Model file for the job. Use its own axes, mm. A direction names the side the tool comes from. Give positions to 0.01 mm unless a question says otherwise; leave off trailing zeros. Loops run counter-clockwise (first coordinate to the right, second up) from the corner with the lowest first, then second, coordinate; pieces in that order, holes last. Notation, with made-up numbers: M -33.75,23.25 L 7.25,23.25 A10 cw 7.25,36.25 Z; hole C 27.5,49 d4. An arc over 180 degrees is marked long. Answer in a Markdown table with one row per item.
```python
from build123d import *

# Parameters (mm, degrees)
F0_R     = 4
F0_R_2   = 1.6
F1_DEPTH = 5
F2_R     = 2


with BuildPart() as f1:
    # F0 (on Front) → F1 (new body)
    with BuildSketch(Plane.XZ):
        with BuildLine():
            Line((10, 57.131427), (-10, 57.131427))
            Line((-10, 57.131427), (-10, 42.131427))
            ThreePointArc((-10, 42.131427), (-7.171573, 40.959855), (-6, 38.131427))
            Line((-6, 38.131427), (-6, 9.131427))
            ThreePointArc((-6, 9.131427), (-7.171573, 6.303), (-10, 5.131427))
            Line((-10, 5.131427), (-10, -1))
            Line((-10, -1), (-3, -8))
            Line((-3, -8), (3, -8))
            Line((3, -8), (10, -1))
            Line((10, -1), (10, 5.131427))
            ThreePointArc((10, 5.131427), (7.171573, 6.303), (6, 9.131427))
            Line((6, 9.131427), (6, 38.131427))
            ThreePointArc((6, 38.131427), (7.171573, 40.959855), (10, 42.131427))
            Line((10, 42.131427), (10, 57.131427))
        make_face()
        Circle(F0_R, mode=Mode.SUBTRACT)
        with Locations((-5.5, 46.631427)):
            Circle(F0_R_2, mode=Mode.SUBTRACT)
        with Locations((-5.5, 52.631427)):
            Circle(F0_R_2, mode=Mode.SUBTRACT)
        with Locations((5.5, 46.631427)):
            Circle(F0_R_2, mode=Mode.SUBTRACT)
        with Locations((5.5, 52.631427)):
            Circle(F0_R_2, mode=Mode.SUBTRACT)
    extrude(amount=F1_DEPTH)

    # F2
    f2_edges = [f1.edges().sort_by_distance(p)[0] for p in [
        (10, -2.5, 57.131427),
        (10, -2.5, 42.131427),
        (-10, -2.5, 42.131427),
        (-10, -2.5, 57.131427),
    ]]
    fillet(f2_edges, radius=F2_R)


solid = f1.part
```
(1) Wall check: L1, parallel to Z at x = 6.5, y = -2.9; L2, parallel to Z at x = -5.75, y = -1.5; L3, parallel to Z at x = -4.25, y = -3.85. Give the ranges that are in metal, low to high.
Established:
| item | result |
|---|---|
| L1 | z = -4.5 to 7.19, 40.07 to 45.38, 47.88 to 51.38, 53.88 to 57.13 |
| L2 | z = -5.25 to 45.05, 48.21 to 51.05, 54.21 to 57.13 |
| L3 | z = -6.75 to 45.63, 47.63 to 51.63, 53.63 to 57.13 |
(2) Saw through at D-D, the plane z = 24.5. Give the cut face in (x, y), and give its area (3 significant figures).
Established:
| item | result |
|---|---|
| outline | M -6,-5 L 6,-5 L 6,0 L -6,0 Z |
| area | 60.0 mm2 |
(3) Which spindle directions (+Z, -Z, +X, -X, +Y, -Y) get a long thin tool onto all of the face, cutting with end or side? Do faces 5 (the cylindrical face through (9.643, -2.535, 42.648)), 6 (the cylindrical face through (-6.754, -2.465, 40.469)), 7 (the flat face through (10, -2, 2)). Say none if no direction does.
Established:
| item | result |
|---|---|
| face 5 | +X, +Y, -Y |
| face 6 | -X, +Y, -Y |
| face 7 | +Z, -Z, +X, +Y, -Y |
(4) Flat gauge pins, fed straight in: P1, Ø1.5, axis at y = -0.5, z = 6.5, coming from the -X side; P2, Ø1.5, axis at y = -3.5, z = 21, coming from the +X side. Where does each tip first touch, or does it go through?
Established:
| item | result |
|---|---|
| P1 | stops at x = -7.86 |
| P2 | stops at x = 6 |
(5) Mould opens along Z. For faces 1 (the cylindrical face through (5.292, -2.465, 54.218)), 2 (the flat face through (0, -2, -8)), 3 (the flat face through (0, 0, 25)), 4 (the flat face through (-6, -2, 24)) say: pulls with the +Z half, pulls with the -Z half, needs draft (parallel to the pull), parting line crosses it, or undercut.
Established:
| item | result |
|---|---|
| face 1 | undercut |
| face 2 | pulls with the -Z half |
| face 3 | needs draft |
| face 4 | undercut |
(6) Saw through at C-C, the plane y = -2.55. Give the cut face in (x, z).
Established:
| item | result |
|---|---|
| outline | M -10,-1 L -3,-8 L 3,-8 L 10,-1 L 10,5.13 A4 cw 6,9.13 L 6,38.13 A4 cw 8.67,41.9 A2 ccw 10,43.79 L 10,55.13 A2 ccw 8,57.13 L -8,57.13 A2 ccw -10,55.13 L -10,43.79 A2 ccw -8.67,41.9 A4 cw -6,38.13 L -6,9.13 A4 cw -10,5.13 Z; hole C -5.5,46.63 d3.2; hole C -5.5,52.63 d3.2; hole C 0,0 d8; hole C 5.5,46.63 d3.2; hole C 5.5,52.63 d3.2 |
(7) Saw through at B-B, the plane x = 0. Give the cut face in (y, z), and give its area (3 significant figures).
Established:
| item | result |
|---|---|
| outline | M -5,-8 L 0,-8 L 0,-4 L -5,-4 Z; M -5,4 L 0,4 L 0,57.13 L -5,57.13 Z |
| area | 286 mm2 |
(8) Saw through at A-A, the plane z = 0. Give the cut face in (x, y).
Established:
| item | result |
|---|---|
| outline | M -10,-5 L -4,-5 L -4,0 L -10,0 Z; M 4,-5 L 10,-5 L 10,0 L 4,0 Z |
